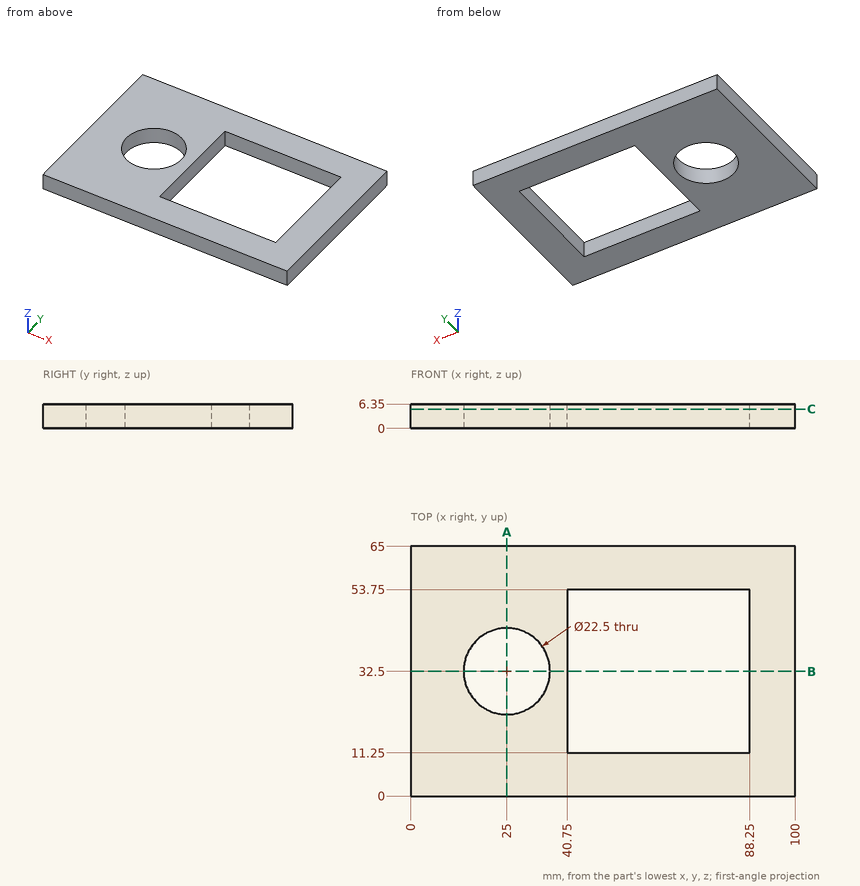
Geometry: see drawing. Coordinates: mm, zero at the bounding-box minimum. Coordinates: 2 decimals unless noted, no trailing zeros. Write each loop counter-clockwise with the first axis right and the second up, starting at its lowest first coordinate (ties: lowest second). Pieces come first, ordered by that corner, then holes. Notation, with made-up numbers: (2.25, 39) - (53.25, 39) arc R22 cw to (53.25, 46) - close; hole circle Ø10 at (73, 48). An arc over 180 degrees is marked (long way). Put each result on its own line as item: value. Start each with the question number.
1) Cut plane B-B (y = 32.5). Return the cut outline in (x, z).
2) Cut plane A-A (x = 25). Return the cut outline in (y, z), plus the area to 3 significant figures.
3) Contact query for a flat-ended pin moving along its axis: pin 1 (13.5 mm diameter, centred on x = 25, y = 32.5, fed in from +Z). Output: stop coordinate, or through.
4) Cut plane C-C (z = 5). Return the cut outline in (x, y).
5) Ray query, L1, parallel to Y at x = 72, z = 5.25; L2, parallel to X at y = 34, z = 5.5; L3, parallel to X at y = 41, z = 4.5. Return the intervals inside material, ascending.
Resolved:
1. outline: (0, 0) - (13.75, 0) - (13.75, 6.35) - (0, 6.35) - close; (36.25, 0) - (40.75, 0) - (40.75, 6.35) - (36.25, 6.35) - close; (88.25, 0) - (100, 0) - (100, 6.35) - (88.25, 6.35) - close
2. outline: (0, 0) - (21.25, 0) - (21.25, 6.35) - (0, 6.35) - close; (43.75, 0) - (65, 0) - (65, 6.35) - (43.75, 6.35) - close
2. area: 270 mm2
3. pin 1: passes through
4. outline: (0, 0) - (100, 0) - (100, 65) - (0, 65) - close; hole circle Ø22.5 at (25, 32.5); hole (40.75, 11.25) - (88.25, 11.25) - (88.25, 53.75) - (40.75, 53.75) - close
5. L1: y = 0 to 11.25, 53.75 to 65
5. L2: x = 0 to 13.85, 36.15 to 40.75, 88.25 to 100
5. L3: x = 0 to 17.63, 32.37 to 40.75, 88.25 to 100
